from build123d import *

# Parameters (mm, degrees)
BASE_FLANGE1_DEPTH           = 2.65684
EDGE_FLANGE1_DEPTH           = 254
EDGE_FLANGE2_STRIP_W         = 16.97736
EDGE_FLANGE2_STRIP_H         = 2.65684
EDGE_FLANGE2_STRIP_CUT_DEPTH = 112.395
EDGE_FLANGE2_DEPTH           = 112.395
EDGE_FLANGE3_DEPTH           = 112.395
EDGE_FLANGE4_DEPTH           = 248.16816
SKETCH22_R                   = 7.14375
CUT_EXTRUDE1_DEPTH           = 2.65684
SKETCH23_R                   = 7.14375
CUT_EXTRUDE2_DEPTH           = 2.65684
SKETCH24_R                   = 7.14375
CUT_EXTRUDE3_DEPTH           = 2.65684


# Sheet-metal steps are written as plain solids
with BuildPart() as part:
    # Sketch1 → Base-Flange1 (new body)
    with BuildSketch(Plane.XY):
        with BuildLine():
            Line((0, 0), (355.6, 0))
            Line((355.6, 0), (355.6, 254))
            Line((355.6, 254), (193.04, 254))
            ThreePointArc((193.04, 254), (177.8, 238.76), (162.56, 254))
            Line((162.56, 254), (0, 254))
            Line((0, 254), (0, 0))
        make_face()
    extrude(amount=-BASE_FLANGE1_DEPTH)

    # Edge-Flange1 section (across the edge) → Edge-Flange1 (add)
    with BuildSketch(Plane(origin=(-3.175, 0, -2.65684), x_dir=(1, 0, 0), z_dir=(0, 1, 0))):
        with BuildLine():
            Line((-2.65684, 3.175), (-2.65684, 115.57))
            Line((-2.65684, 115.57), (0, 115.57))
            Line((0, 115.57), (0, 3.175))
            ThreePointArc((0, 3.175), (0.92993597, 0.92993597), (3.175, 0))
            Line((3.175, 0), (3.175, -2.65684))
            ThreePointArc((3.175, -2.65684), (-0.948733611, -0.948733611), (-2.65684, 3.175))
        make_face()
    extrude(amount=EDGE_FLANGE1_DEPTH)

    # Edge-Flange2 strip (across the edge) → Edge-Flange2 strip cut (cut)
    with BuildSketch(Plane(origin=(-5.83184, 254, -5.83184), x_dir=(0, -1, 0), z_dir=(0, 0, -1))):
        with Locations((-2.65684, -1.32842)):
            Rectangle(EDGE_FLANGE2_STRIP_W, EDGE_FLANGE2_STRIP_H)
    extrude(amount=EDGE_FLANGE2_STRIP_CUT_DEPTH, mode=Mode.SUBTRACT)

    # Edge-Flange2 section (across the edge) → Edge-Flange2 (add)
    with BuildSketch(Plane(origin=(-5.83184, 254, -5.83184), x_dir=(0, -1, 0), z_dir=(0, 0, -1))):
        with BuildLine():
            Line((0, 3.175), (0, 57.15))
            Line((0, 57.15), (2.65684, 57.15))
            Line((2.65684, 57.15), (2.65684, 3.175))
            ThreePointArc((2.65684, 3.175), (3.58677597, 0.92993597), (5.83184, 0))
            Line((5.83184, 0), (5.83184, -2.65684))
            ThreePointArc((5.83184, -2.65684), (1.708106389, -0.948733611), (0, 3.175))
        make_face()
    extrude(amount=EDGE_FLANGE2_DEPTH)

    # Edge-Flange3 section (across the edge) → Edge-Flange3 (add)
    with BuildSketch(Plane(origin=(-5.83184, -3.175, -118.22684), x_dir=(0, 1, 0), z_dir=(0, 0, 1))):
        with BuildLine():
            Line((-2.65684, 3.175), (-2.65684, 57.15))
            Line((-2.65684, 57.15), (0, 57.15))
            Line((0, 57.15), (0, 3.175))
            ThreePointArc((0, 3.175), (0.92993597, 0.92993597), (3.175, 0))
            Line((3.175, 0), (3.175, -2.65684))
            ThreePointArc((3.175, -2.65684), (-0.948733611, -0.948733611), (-2.65684, 3.175))
        make_face()
    extrude(amount=EDGE_FLANGE3_DEPTH)

    # Edge-Flange4 section (across the edge) → Edge-Flange4 (add)
    with BuildSketch(Plane(origin=(-3.175, 0, -121.40184), x_dir=(0, 0, 1), z_dir=(0, 1, 0))):
        with BuildLine():
            Line((-2.65684, 3.175), (-2.65684, 25.4))
            Line((-2.65684, 25.4), (0, 25.4))
            Line((0, 25.4), (0, 3.175))
            ThreePointArc((0, 3.175), (0.92993597, 0.92993597), (3.175, 0))
            Line((3.175, 0), (3.175, -2.65684))
            ThreePointArc((3.175, -2.65684), (-0.948733611, -0.948733611), (-2.65684, 3.175))
        make_face()
    extrude(amount=EDGE_FLANGE4_DEPTH)

    # Sketch22 → Cut-Extrude1 (cut)
    with BuildSketch(Plane(origin=(0, 254, 0), x_dir=(1, 0, 0), z_dir=(0, 1, 0))):
        with Locations(Location((-40.76446, 86.995, 0), (0, 0, 180))):
            Circle(SKETCH22_R)
        with Locations(Location((-40.76446, 36.195, 0), (0, 0, 180))):
            Circle(SKETCH22_R)
    extrude(amount=-CUT_EXTRUDE1_DEPTH, mode=Mode.SUBTRACT)

    # Sketch23 → Cut-Extrude2 (cut)
    with BuildSketch(Plane(origin=(0, -3.175, 0), x_dir=(1, 0, 0), z_dir=(0, 1, 0))):
        with Locations(Location((-34.40684, 86.36, 0), (0, 0, 180))):
            Circle(SKETCH23_R)
        with Locations(Location((-34.40684, 35.56, 0), (0, 0, 180))):
            Circle(SKETCH23_R)
    extrude(amount=-CUT_EXTRUDE2_DEPTH, mode=Mode.SUBTRACT)

    # Sketch24 → Cut-Extrude3 (cut)
    with BuildSketch(Plane.ZY.offset(5.83184)):
        with Locations((-86.995, 41.79316)):
            Circle(SKETCH24_R)
        with Locations((-34.40684, 41.79316)):
            Circle(SKETCH24_R)
    extrude(amount=-CUT_EXTRUDE3_DEPTH, mode=Mode.SUBTRACT)


solid = part.part
Could you check a few things on this model? Use its own coordinates, in mm. A direction names the side the tool comes from. Give positions to 0.01 mm unless a question says otherwise; leave off trailing zeros. Loops run counter-clockwise (first coordinate to the right, second up) from the corner with the lowest first, then second, coordinate; pieces in that order, holes last. Notation, with made-up numbers: M 55.5,4 L 101.5,4 A20 ccw 101.5,33 Z; hole C 6.25,36.25 d1. An arc over 180 degrees is marked long. Answer as a JSON object with one key per item and string values.
Q1. For faces 4 (the flat face through (-36, -3.175, -63)), 5 (the flat face through (11, 122, -121.402)), 6 (the cylindrical face through (-39.22, 252.69, -43.17)), 7 (the cylindrical face through (-32.858, -4.485, -93.334)), which set-ups out of +Z, -Z, +X, -X, +Y, -Y let a thin tool reach every point of the face, with its end or its side?
Values found:
{"face 4": "+Z, -Z, -X", "face 5": "+X, +Y, -Y", "face 6": "+Y", "face 7": "-Y"}
Q2. Suppose I cut it at D-D, the plane x = 177.8. List the corners of the cut face in (y, z) for me.
Values found:
{"outline": "M 0,-2.66 L 238.76,-2.66 L 238.76,0 L 0,0 Z"}
Q3. Suppose I cut it at C-C, the plane x = 102. List the corners of the cut face in (y, z) for me, plus the area to 3 significant figures.
Values found:
{"outline": "M 0,-2.66 L 254,-2.66 L 254,0 L 0,0 Z", "area": "675 mm²"}
Q4. Suppose I cut it at B-B, the plane y = 13.5. List the corners of the cut face in (x, z) for me (3 decimals).
Values found:
{"outline": "M -5.832,-118.227 A5.832 ccw 0,-124.059 L 22.225,-124.059 L 22.225,-121.402 L 0,-121.402 A3.175 cw -3.175,-118.227 L -3.175,-5.832 A3.175 cw 0,-2.657 L 355.6,-2.657 L 355.6,0 L 0,0 A5.832 ccw -5.832,-5.832 Z"}
Q5. Suppose I cut it at A-A, the plane z = -99.5. List the corners of the cut face in (x, y) for me (3 decimals), plus the area to 3 significant figures.
Values found:
{"outline": "M -62.982,-5.832 L -9.007,-5.832 A5.832 ccw -3.175,0 L -3.175,248.168 A5.832 ccw -9.007,254 L -62.982,254 L -62.982,251.343 L -9.007,251.343 A3.175 cw -5.832,248.168 L -5.832,0 A3.175 cw -9.007,-3.175 L -62.982,-3.175 Z", "area": "984 mm²"}
Q6. If I drill on probe 1 along X at (y, z) = (106.5, -23.5) (3 decimals); probe 2 along Z at (x, y) = (248.5, 175.5); probe 3 along Y at (x, z) = (-15, -107.5) (3 decimals), over which ranges is the centre line in solid material (lowest first)? Write a range as [from, to].
Values found:
{"probe 1": "x = [-5.832, -3.175]", "probe 2": "z = [-2.66, 0]", "probe 3": "y = [-5.832, -3.175], [251.343, 254]"}
Q7. For P1, Ø6, axis at x = 227, y = 144, coming from the -Z side; P2, Ø1, axis at y = 201, z = -31, coming from the -X side; P3, Ø1.3, axis at x = -4, y = 250.5, coming from the -Z side; P4, Ø11.5, axis at y = 41.79, z = -87, coming from the +X side, each with a flat end and sliding along its axis, tell me the tip position at first contact or that it passes through.
Values found:
{"P1": "stops at z = -2.66", "P2": "stops at x = -5.83", "P3": "stops at z = -118.23", "P4": "passes through"}
Q8. If we mould it in two halves opening along Y, with no side actions, what happens to faces 1 (the flat face through (-36, -5.832, -63)), 2 (the cylindrical face through (-4.522, 48.876, -35.337)), 3 (the flat face through (175, 129, 0))? For each: pulls with the +Y half, pulls with the -Y half, needs draft (parallel to the pull), parting line crosses it, or undercut.
Values found:
{"face 1": "pulls with the -Y half", "face 2": "undercut", "face 3": "needs draft"}
